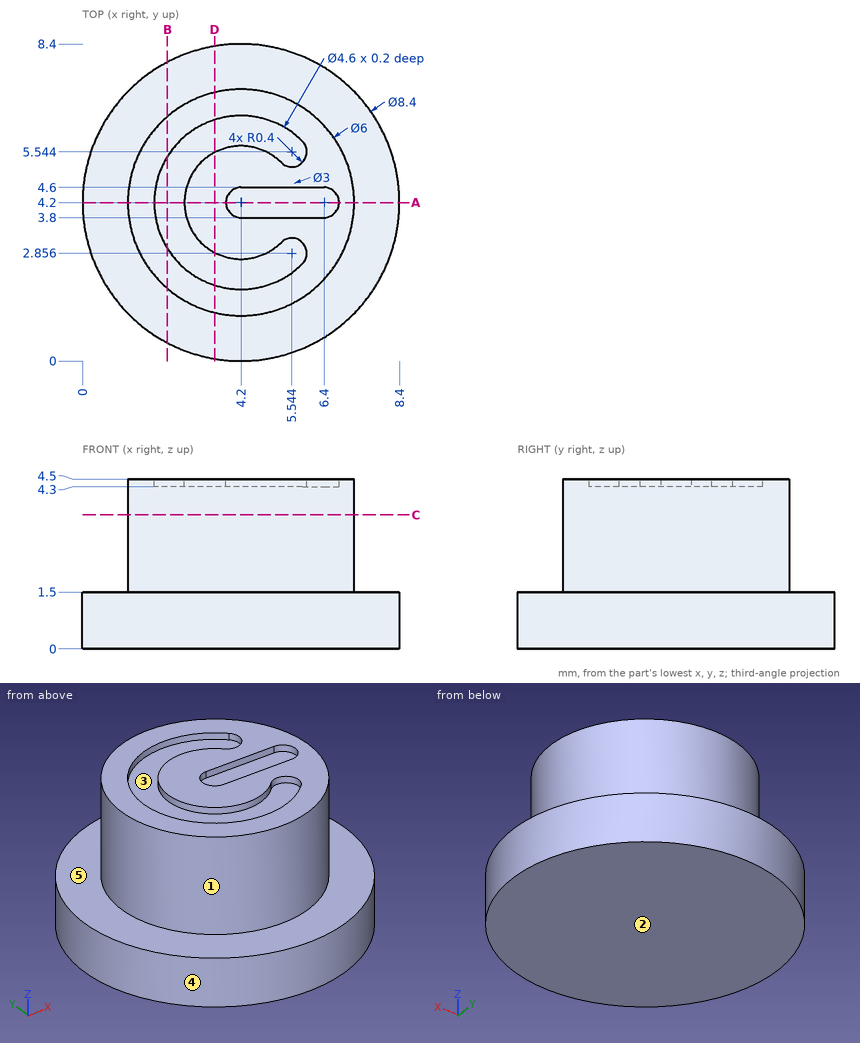
Geometry: see drawing. Coordinates: mm, zero at the bounding-box minimum. A direction names the side the tool comes from. Round coordinates to 2 decimals unless told otherwise and drop trailing zeros. Loops run counter-clockwise (first coordinate to the right, second up) from the corner with the lowest first, then second, coordinate; pieces in that order, holes last. Notation, with made-up numbers: (61, -34.5) -> (109, -34.5) arc R31 ccw to (109, -5.5) -> close; hole circle Ø6 at (86.5, 47). An arc over 180 degrees is marked (long way). Write each question's results on one line, items separated by ' | '.
Item 1: Pull-direction query (Y, two-part tool) for the marked faces 3, 4 and 5; classes: pulls with the +Y half, pulls with the -Y half, needs draft (parallel to the pull), parting line crosses it, or undercut.
Answers below:
face 3: undercut | face 4: parting line crosses it | face 5: needs draft
Item 2: Line query: probe 1 along Y at (x, z) = (4.2, 4.4); probe 2 along Z at (x, y) = (7.75, 5.5); probe 3 along Z at (x, y) = (2.5, 3.75). Output: solid intervals per line, ascending. Write a range as [from, to].
Answers below:
probe 1: y = [1.2, 1.9], [2.7, 3.8], [4.6, 5.7], [6.5, 7.2] | probe 2: z = [0, 1.5] | probe 3: z = [0, 4.3]
Item 3: Cut plane D-D on x = 3.5. Return the cut outline in (y, z), and give its area (3 significant figures).
Answers below:
outline: (0.06, 0) -> (8.34, 0) -> (8.34, 1.5) -> (7.12, 1.5) -> (7.12, 4.5) -> (6.39, 4.5) -> (6.39, 4.3) -> (5.53, 4.3) -> (5.53, 4.5) -> (2.87, 4.5) -> (2.87, 4.3) -> (2.01, 4.3) -> (2.01, 4.5) -> (1.28, 4.5) -> (1.28, 1.5) -> (0.06, 1.5) -> close | area: 29.6 mm²
Item 4: Cut plane B-B on x = 2.25. Return the cut outline in (y, z).
Answers below:
outline: (0.48, 0) -> (7.92, 0) -> (7.92, 1.5) -> (6.48, 1.5) -> (6.48, 4.5) -> (5.42, 4.5) -> (5.42, 4.3) -> (2.98, 4.3) -> (2.98, 4.5) -> (1.92, 4.5) -> (1.92, 1.5) -> (0.48, 1.5) -> close
Item 5: Cut plane C-C on z = 3.55. Return the cut outline in (x, y), and give its area (3 significant figures).
Answers below:
outline: circle Ø6 at (4.2, 4.2) | area: 28.3 mm²
Item 6: Set-up query: the marked faces 1 and 2. Return all of +Z, -Z, +X, -X, +Y, -Y with unobstructed straight access to the full face (end or side cutting, diameter ignored); none if empty.
Answers below:
face 1: +Z | face 2: -Z, +X, -X, +Y, -Y
Item 7: Pin query (flat end, axial travel): pin 1 Ø2 at (y, z) = (5.5, 2) entering from +X; pin 2 Ø3 at (x, y) = (4.2, 4.2) entering from +Z; pin 3 Ø1.5 at (x, z) = (7.5, 3.5) entering from -Y. Return the tip coordinate at first contact, or that it passes through.
Answers below:
pin 1: stops at x = 8.38 | pin 2: stops at z = 4.5 | pin 3: stops at y = 2.62
Item 8: Cut plane A-A on y = 4.2. Return the cut outline in (x, z).
Answers below:
outline: (0, 0) -> (8.4, 0) -> (8.4, 1.5) -> (7.2, 1.5) -> (7.2, 4.5) -> (6.8, 4.5) -> (6.8, 4.3) -> (3.8, 4.3) -> (3.8, 4.5) -> (2.7, 4.5) -> (2.7, 4.3) -> (1.9, 4.3) -> (1.9, 4.5) -> (1.2, 4.5) -> (1.2, 1.5) -> (0, 1.5) -> close
